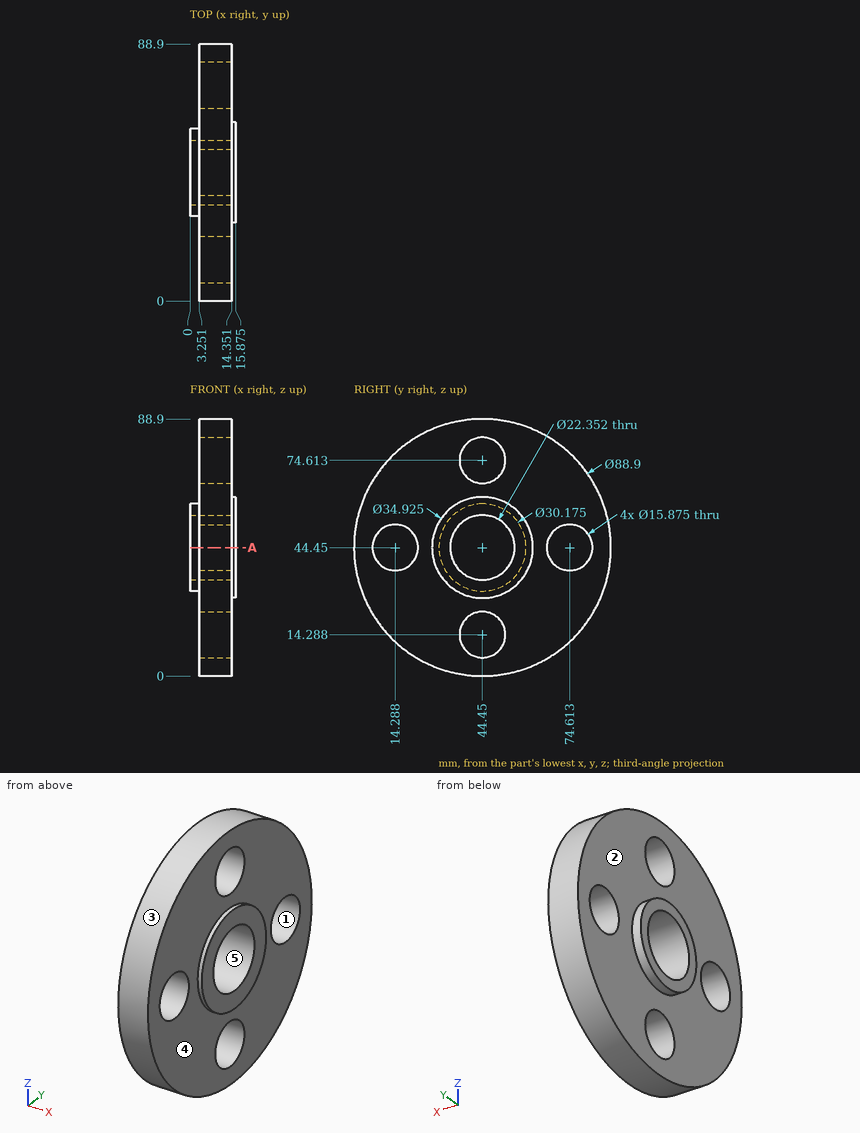
Geometry check sheet. Reference: drawing and pictorial views, mm from the part's lowest x, y, z. A direction names the side the tool comes from. Give positions to 0.01 mm unless a question says otherwise; leave off trailing zeros. Use CSV: the item, a comma, the result in double quotes. Start each with the question number.
Q1. Scan lines: probe 1 along X at (y, z) = (41, 26.5); probe 2 along Z at (x, y) = (6, 39.5) (1 decimal); probe 3 along Z at (x, y) = (12.5, 11) (1 decimal). Record each from-to range of solid material in increasing order. Write a range as from..to.
Q2. Access from +Z, -Z, +X, -X, +Y, -Y to the whole of each face (thin tool, end or side, straight path). Record for the marked faces 4 and 5.
Q3. Go/stop test with flat-tipped pins: pin 1 Ø18.5 at (y, z) = (14.29, 44.45) entering from -X; pin 2 Ø1 at (x, y) = (11.5, 34.5) entering from +Z; pin 3 Ø12 at (y, z) = (30.5, 78.5) entering from +X; pin 4 Ø14.5 at (y, z) = (74.61, 44.45) entering from +X. Record where each tip stops, or that it passes through.
Q4. Section check A-A, the plane z = 44.45. Count the separate pieces of the cut face and the enclosed holes in it, and give its area (3 significant figures).
Q5. Release check for a two-part mould opening along Y. For the marked faces 1, 2 and 3 record: +Y half, -Y half, draft (parallel to the pull), parting line (faces both ways), or undercut.
Findings below:
1,probe 1,"x = 3.25..14.35"
1,probe 2,"z = 0.3..8.1, 20.5..34.4, 54.5..68.4, 80.8..88.6"
1,probe 3,"z = 15.2..37.2, 51.7..73.7"
2,face 4,"+X"
2,face 5,"+X, -X"
3,pin 1,"stops at x = 3.25"
3,pin 2,"stops at z = 87.88"
3,pin 3,"stops at x = 14.35"
3,pin 4,"passes through"
4,separate pieces,"4"
4,enclosed holes,"0"
4,area,"431 mm^2"
5,face 1,"undercut"
5,face 2,"draft"
5,face 3,"parting line"
